Check sheet for the drawn part. Datum: minimum x, y, z corner. Units: mm. Coordinates: 2 decimals unless noted, no trailing zeros. Loops run counter-clockwise (first coordinate to the right, second up) from the corner with the lowest first, then second, coordinate; pieces in that order, holes last. Notation, with made-up numbers: M 3,48.25 L 62,48.25 A4 cw 62,52.25 Z; hole C 62.25,67 d9. An arc over 180 degrees is marked long. Use CSV: the item, a comma, the result in double quotes. Start each with the question number.
(1) Section check A-A on z = 1. Give the number of separate pieces and of enclosed holes in the cut face, and give its area (3 significant figures).
(2) Section check C-C on x = 22. Record the cut outline in (y, z) (1 decimal).
(3) Scan lines: line 1 (X direction, y = 6, z = 1.55); line 2 (Y direction, x = 31.5, z = 2.3) (1 decimal); line 3 (Y direction, x = 33, z = 2.6) (1 decimal). Record each from-to range of solid material in increasing order.
(4) Section check B-B on y = 17. Record the cut outline in (x, z) (1 decimal).
(5) Draft check along Z on the marked faces 1 and 2. Enter one of: pulls with the +Z half, pulls with the -Z half, needs draft (parallel to the pull), parting line crosses it, or undercut.
(6) Go/stop test with flat-tipped pins: pin 1 Ø1.5 at (y, z) = (29, 2.5) entering from -X; pin 2 Ø0.7 at (x, z) = (30.5, 1.5) entering from +Y (3 decimals); pin 3 Ø8 at (x, y) = (64.5, 14) entering from -Z. Record where each tip stops, or that it passes through.
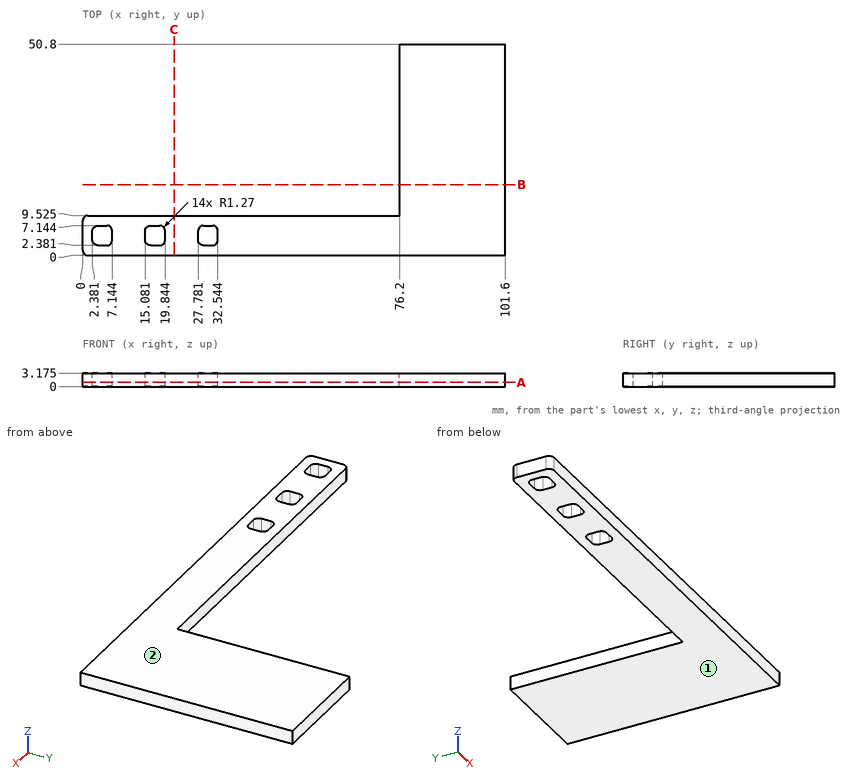
Outcome:
1,separate pieces,"1"
1,enclosed holes,"3"
1,area,"1,950 mm²"
2,outline,"M 0,0 L 9.5,0 L 9.5,3.2 L 0,3.2 Z"
3,line 1,"x = 0 to 2.39, 7.14 to 15.09, 19.84 to 27.79, 32.54 to 101.6"
3,line 2,"y = 0 to 2.4, 7.1 to 9.5"
3,line 3,"y = 0 to 9.5"
4,outline,"M 76.2,0 L 101.6,0 L 101.6,3.2 L 76.2,3.2 Z"
5,face 1,"pulls with the -Z half"
5,face 2,"pulls with the +Z half"
6,pin 1,"stops at x = 76.2"
6,pin 2,"stops at y = 9.525"
6,pin 3,"passes through"
